Could you check a few things on this model? Use its own coordinates, in mm. Give positions to 0.01 mm unless a question says otherwise; leave off trailing zeros. Order: outer loops, then holes, each group sorted by start corner. A loop starts at its lowest first (then second) coordinate and runs counter-clockwise, first axis right, second up.
from build123d import *

# Parameters (mm, degrees)
SKETCH002_R        = 16.6
PAD001_DEPTH       = 14.2
SKETCH003_R        = 16.6
SKETCH003_R_2      = 13.25
POCKET001_DEPTH    = 2.6
SKETCH009_R        = 4
POCKET004_DEPTH    = 2
SKETCH005_R        = 1.6
PAD005_DEPTH       = 2.3
BODY001_ROLL_ANGLE = -0.43547


with BuildPart() as part:
    # Sketch002 → Pad001 (new body)
    with BuildSketch(Plane.XZ):
        Circle(SKETCH002_R)
    extrude(amount=PAD001_DEPTH)

    # Sketch003 → Pocket001 (cut)
    with BuildSketch(Plane.XZ):
        Circle(SKETCH003_R)
        Circle(SKETCH003_R_2, mode=Mode.SUBTRACT)
    extrude(amount=POCKET001_DEPTH, mode=Mode.SUBTRACT)

    # Sketch009 (on Face3 of Pocket001) → Pocket004 (cut)
    with BuildSketch(Plane.XZ.offset(14.2)):
        with Locations((0, 8)):
            Circle(SKETCH009_R)
    extrude(amount=-POCKET004_DEPTH, mode=Mode.SUBTRACT)

    # Sketch005 (on Face3 of Pocket001) → Pad005 (join)
    with BuildSketch(Plane.XZ.offset(14.2)):
        with BuildLine():
            ThreePointArc((19.2, -4.1), (23.300001, 0), (19.2, 4.1))
            Line((19.2, 4.1), (9.6, 4.1))
            Line((9.6, 4.1), (9.6, -4.1))
            Line((9.6, -4.1), (19.2, -4.1))
        make_face()
        with Locations((19.200001, 0)):
            Circle(SKETCH005_R, mode=Mode.SUBTRACT)
    pad005 = extrude(amount=-PAD005_DEPTH)

    # Mirrored: Pad005 across Sketch005 V_Axis
    add(pad005.mirror(Plane(origin=(0, -14.2, 0), x_dir=(0, -1, 0), z_dir=(1, 0, 0))))


with BuildPart() as part_1:
    # Body001 roll: moved
    add(part.part.rotate(Axis((0, 0, 0), (1, 0, 0)), BODY001_ROLL_ANGLE))


with BuildPart() as part_2:
    # Body001 placement: moved
    add(part_1.part.moved(Location((0, 0, 0))))


solid = part_2.part
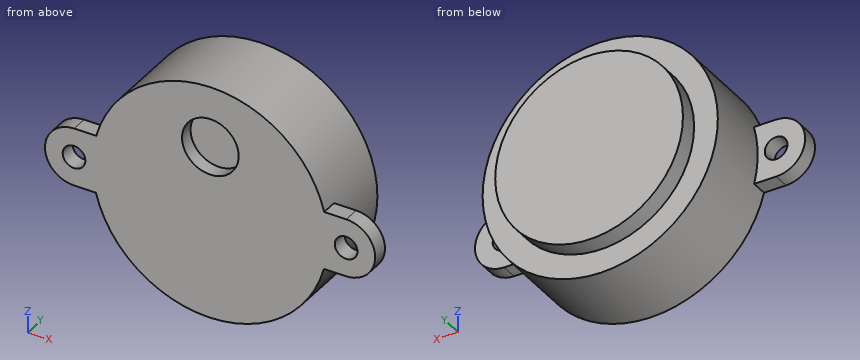
Item 1: Imagine slicing it at D-D on x = -7. List the corners of the cut face in (y, z) for me, then the cut area to 3 significant figures.
Findings:
outline: (-14.31, -14.94) - (-2.71, -15.03) - (-2.69, -11.23) - (-0.09, -11.25) - (0.09, 11.25) - (-2.51, 11.27) - (-2.49, 15.07) - (-14.09, 15.16) - close
area: 408 mm2
Item 2: Imagine slicing it at A-A on x = 20. List the corners of the cut face in (y, z) for me, then the cut area to 3 significant figures.
Findings:
outline: (-14.23, -3.91) - (-11.93, -3.93) - (-11.91, -1.3) - (-14.21, -1.28) - close; (-14.19, 1.49) - (-11.89, 1.48) - (-11.87, 4.11) - (-14.17, 4.13) - close
area: 12.1 mm2
Item 3: Imagine slicing it at C-C on z = -0.5. Give the number of separate pieces and of enclosed holes in the cut face, then the cut area to 3 significant figures.
Findings:
separate pieces: 3
enclosed holes: 0
area: 471 mm2
Item 4: Imagine slicing it at B-B on x = 11. List the corners of the cut face in (y, z) for me, then the cut area to 3 significant figures.
Findings:
outline: (-14.29, -12.32) - (-2.69, -12.41) - (-2.66, -7.37) - (-0.06, -7.39) - (0.06, 7.39) - (-2.54, 7.41) - (-2.51, 12.45) - (-14.11, 12.54) - close
area: 327 mm2
Item 5: Please list where these lines run through material, in increasing order: line 1 along Z through (x, y) = (-20, -12.75); line 2 along X through (y, z) = (-7, -11.5); line 3 along Y through (x, z) = (6, 2.5).
Findings:
line 1: z = -3.92 to -1.29, 1.48 to 4.12
line 2: x = -11.92 to 11.92
line 3: y = -14.18 to 0.02
Item 6: For pin 1 (3 mm diameter, centred on x = -1, z = -10.5, fed in from -Y); pin 2 (2 mm diameter, centred on y = -1.5, z = -8, fed in from -X); pin 3 (1 mm diameter, centred on y = -12.5, z = 7, fed in from +X), each with a flat end and sliding along its axis, tell me the tip position at first contact or that it passes through.
Findings:
pin 1: stops at y = -14.29
pin 2: stops at x = -11.24
pin 3: stops at x = 15.31
